from build123d import *

# Parameters (mm, degrees)
SKETCH2_R           = 37.5
SKETCH2_R_2         = 5.35
BOSS_EXTRUDE2_DEPTH = 8
SKETCH14_R          = 2
CUT_EXTRUDE6_DEPTH  = 54.633012222
SKETCH3_R           = 20.71
SKETCH3_R_2         = 19.21
CUT_EXTRUDE2_DEPTH  = 2
SKETCH7_R           = 12.5
SKETCH7_R_2         = 10.5
BOSS_EXTRUDE4_DEPTH = 80
SKETCH10_R          = 12.5
BOSS_EXTRUDE5_DEPTH = 2.01
BOSS_EXTRUDE5_DRAFT = -75
SKETCH11_R          = 10.5
CUT_EXTRUDE3_DEPTH  = 105.4715277
BOSS_EXTRUDE6_START = 3
SKETCH12_R          = 20.001422123
SKETCH12_R_2        = 10.5
BOSS_EXTRUDE6_DEPTH = 3
SKETCH13_R          = 13.1
CUT_EXTRUDE4_DEPTH  = 2.5
CHAMFER1_SIZE       = 10


with BuildPart() as part:
    # Sketch2 → Boss-Extrude2 (new body)
    with BuildSketch(Plane.XY):
        Circle(SKETCH2_R)
        Circle(SKETCH2_R_2, mode=Mode.SUBTRACT)
    extrude(amount=BOSS_EXTRUDE2_DEPTH)

    # Sketch14 → Cut-Extrude6 (cut, through all)
    with BuildSketch(Plane.XY):
        with Locations((0, 33.75)):
            Circle(SKETCH14_R)
        with Locations((-23.864853865, 23.864853865)):
            Circle(SKETCH14_R)
        with Locations((-33.75, 0)):
            Circle(SKETCH14_R)
        with Locations((-23.864853865, -23.864853865)):
            Circle(SKETCH14_R)
        with Locations((0, -33.75)):
            Circle(SKETCH14_R)
        with Locations((23.864853865, -23.864853865)):
            Circle(SKETCH14_R)
        with Locations((33.75, 0)):
            Circle(SKETCH14_R)
        with Locations((23.864853865, 23.864853865)):
            Circle(SKETCH14_R)
    extrude(amount=CUT_EXTRUDE6_DEPTH, mode=Mode.SUBTRACT)

    # Sketch3 → Cut-Extrude2 (cut)
    with BuildSketch(Plane.XY):
        Circle(SKETCH3_R)
        Circle(SKETCH3_R_2, mode=Mode.SUBTRACT)
    extrude(amount=CUT_EXTRUDE2_DEPTH, mode=Mode.SUBTRACT)

    # Sketch7 → Boss-Extrude4 (add)
    with BuildSketch(Plane.XY.offset(8)):
        Circle(SKETCH7_R)
        Circle(SKETCH7_R_2, mode=Mode.SUBTRACT)
    extrude(amount=BOSS_EXTRUDE4_DEPTH)


with BuildPart() as boss_extrude5_tool:
    # Sketch10 → Boss-Extrude5 (with draft: the straight prism first)
    with BuildSketch(Plane.XY.offset(88)):
        Circle(SKETCH10_R)
    extrude(amount=BOSS_EXTRUDE5_DEPTH)
    # Boss-Extrude5: the draft: its side faces are tilted about the plane it starts from
    boss_extrude5_sides = [boss_extrude5_tool.faces().sort_by_distance(p)[0] for p in [
        (-12.5, 0, 89.005),
    ]]
    draft(boss_extrude5_sides, Plane.XY.offset(88), BOSS_EXTRUDE5_DRAFT)


with BuildPart() as part_1:
    add(part.part)

    # Boss-Extrude5: add boss_extrude5_tool
    add(boss_extrude5_tool.part)

    # Sketch11 → Cut-Extrude3 (cut, through all)
    with BuildSketch(Plane.XY.offset(90.01)):
        Circle(SKETCH11_R)
    extrude(amount=-CUT_EXTRUDE3_DEPTH, mode=Mode.SUBTRACT)

    # Sketch12 → Boss-Extrude6 (add)
    with BuildSketch(Plane.XY.offset(90.01).offset(BOSS_EXTRUDE6_START)):
        Circle(SKETCH12_R)
        Circle(SKETCH12_R_2, mode=Mode.SUBTRACT)
    extrude(amount=-BOSS_EXTRUDE6_DEPTH)

    # Sketch13 → Cut-Extrude4 (cut)
    with BuildSketch(Plane.XY.offset(93.01)):
        Circle(SKETCH13_R)
    extrude(amount=-CUT_EXTRUDE4_DEPTH, mode=Mode.SUBTRACT)

    # Chamfer1
    chamfer1_edges = [part_1.edges().sort_by_distance(p)[0] for p in [
        (-12.5, 0, 8),
    ]]
    chamfer(chamfer1_edges, length=CHAMFER1_SIZE)


solid = part_1.part
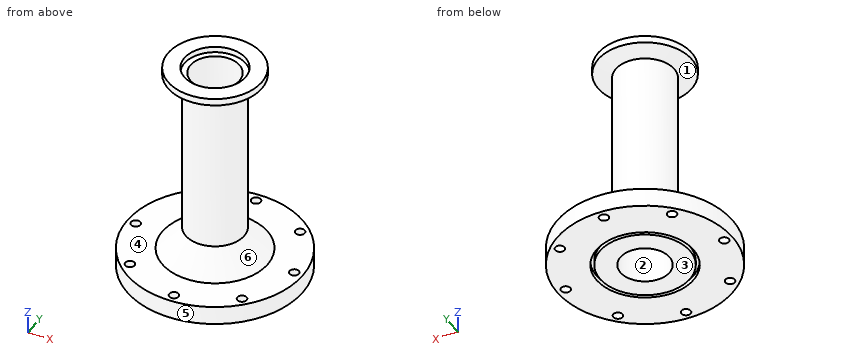
Here's how the part is built. I have some questions about the finished solid (model axes, mm). Face numbers are marked on the shaded views. A direction names the side the tool comes from. Coordinates: 2 decimals unless noted, no trailing zeros. Loops run counter-clockwise (first coordinate to the right, second up) from the corner with the lowest first, then second, coordinate; pieces in that order, holes last.
1. For P1, Ø5, axis at y = -13, z = 61, coming from the +X side; P2, Ø4.5, axis at x = 23.86, y = 23.86, coming from the -Z side; P3, Ø2, axis at y = -0.5, z = 74.5, coming from the +X side; P4, Ø5, axis at y = 1, z = 27.5, coming from the -X side, each with a flat end and sliding along its axis, tell me the tip position at first contact or that it passes through.
2. For the marked faces 4, 5 and 6, which set-ups out of +Z, -Z, +X, -X, +Y, -Y let a thin tool reach every point of the face, with its end or its side?
3. Imagine slicing it at D-D, the plane y = 0. Count the separate pieces of the cut face and the enclosed holes in it, and give its area (3 significant figures).
4. Imagine slicing it at A-A, the plane y = 33.75. Please give me the cut outline in (x, z), and give its area (3 significant figures).
5. I need wall thicknesses on L1, parallel to Z at x = -17, y = 19; L2, parallel to Y at x = -1.5, z = 75.5; L3, parallel to X at y = -9.5, z = 73.5. Which ranges of each line are inside material? Lowest first, please.
6. If we mould it in two halves opening along X, with no side actions, what happens to the marked faces 1, 2 and 3? For each: pulls with the +X half, pulls with the -X half, needs draft (parallel to the pull), parting line crosses it, or undercut.
7. Imagine slicing it at C-C, the plane z = 57. Please give me the cut outline in (x, y), and give its area (3 significant figures).
Taken from the geometry:
1. P1: stops at x = 6.78
1. P2: stops at z = 0
1. P3: stops at x = 12.5
1. P4: stops at x = -12.5
2. face 4: +Z
2. face 5: +Z, -Z
2. face 6: none
3. separate pieces: 4
3. enclosed holes: 0
3. area: 849 mm2
4. outline: (-16.35, 0) - (-2, 0) - (-2, 8) - (-16.35, 8) - close; (2, 0) - (16.35, 0) - (16.35, 8) - (2, 8) - close
4. area: 230 mm2
5. L1: z = 0 to 8
5. L2: y = -12.41 to -10.39, 10.39 to 12.41
5. L3: x = -8.12 to -4.47, 4.47 to 8.12
6. face 1: parting line crosses it
6. face 2: undercut
6. face 3: needs draft
7. outline: circle Ø25 at (0, 0); hole circle Ø21 at (0, 0)
7. area: 145 mm2
